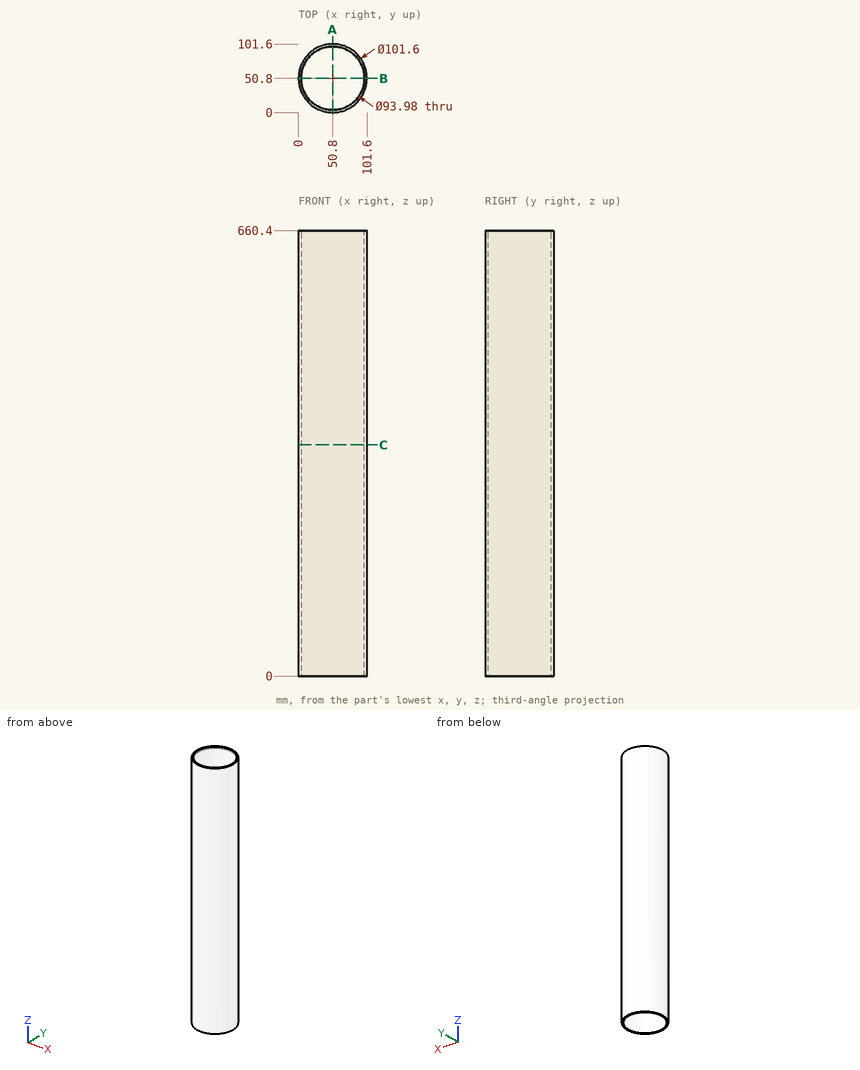
Input: dimensioned drawing with shaded views. Units: mm. Origin: part minimum x, y, z. Round coordinates to 2 decimals unless told otherwise and drop trailing zeros. Loops run counter-clockwise (first coordinate to the right, second up) from the corner with the lowest first, then second, coordinate; pieces in that order, holes last. Notation, with made-up numbers: (53, -3) -> (99, -3) arc R25 cw to (99, 17) -> close; hole circle Ø8 at (-12, -38.75). An arc over 180 degrees is marked (long way). Answer as a JSON object with one key per item and string values. Group by question number.
Q1. Contact query for flat-ended pins moving along their axis: P1, Ø4, axis at x = 58.5, z = 519.5, coming from the +Y side; P2, Ø2, axis at y = 47.5, z = 86.5, coming from the +X side; P3, Ø8, axis at y = 34.5, z = 159.5, coming from the -X side. Output: stop coordinate, or through.
Q2. Section query A-A (x = 50.8). Output: boundary loops of the cut face in (y, z).
Q3. Ray query, line 1 (Y direction, x = 50, z = 240); line 2 (X direction, y = 47.5, z = 417.5); line 3 (X direction, y = 15, z = 523). Return the intervals inside material, ascending. Write a range as from..to.
Q4. Section query C-C (z = 342.5). Output: boundary loops of the cut face in (x, y).
Completed:
{
 "1": {"P1": "y = 101.28", "P2": "x = 101.55", "P3": "x = 1.51"},
 "2": {"outline": "(0, 0) -> (3.81, 0) -> (3.81, 660.4) -> (0, 660.4) -> close; (97.79, 0) -> (101.6, 0) -> (101.6, 660.4) -> (97.79, 660.4) -> close"},
 "3": {"line 1": "0.01..3.82, 97.78..101.59", "line 2": "0.11..3.93, 97.67..101.49", "line 3": "14.76..20.36, 81.24..86.84"},
 "4": {"outline": "circle Ø101.6 at (50.8, 50.8); hole circle Ø93.98 at (50.8, 50.8)"}
}
